from build123d import *

# Parameters (mm, degrees)
SKETCH1_W               = 74.5
SKETCH1_H               = 30
BOSS_EXTRUDE1_DEPTH     = 2
SKETCH4_W               = 2
SKETCH4_H               = 30
BOSS_EXTRUDE2_DEPTH     = 5
CUT_EXTRUDE1_DEPTH      = 41.268629229
CUT_EXTRUDE1_DEPTH_BACK = 41.268629229
SKETCH5_W               = 2
SKETCH5_H               = 15
CUT_EXTRUDE2_DEPTH      = 41.268629229
CUT_EXTRUDE2_DEPTH_BACK = 41.268629229
SKETCH6_R               = 7.5
FILLET1_R               = 1


with BuildPart() as part:
    # Sketch1 → Boss-Extrude1 (new body)
    with BuildSketch(Plane(origin=(0, 0, 0), x_dir=(1, 0, 0), z_dir=(0, 1, 0))):
        Rectangle(SKETCH1_W, SKETCH1_H)
    extrude(amount=BOSS_EXTRUDE1_DEPTH)

    # Sketch4 → Boss-Extrude2 (add)
    with BuildSketch(Plane(origin=(0, 0, 0), x_dir=(1, 0, 0), z_dir=(0, 1, 0))):
        with Locations((36.25, 0)):
            Rectangle(SKETCH4_W, SKETCH4_H)
        with Locations((-36.25, 0)):
            Rectangle(SKETCH4_W, SKETCH4_H)
    extrude(amount=BOSS_EXTRUDE2_DEPTH)

    # Sketch5 → Cut-Extrude1 (cut, two sides: drawn at the far end of the back side and taken through both)
    with BuildSketch(Plane(origin=(0, 2, 0), x_dir=(1, 0, 0), z_dir=(0, 1, 0)).offset(-CUT_EXTRUDE1_DEPTH_BACK)):
        with Locations((0, -7.5)):
            Rectangle(SKETCH5_W, SKETCH5_H)
    extrude(amount=CUT_EXTRUDE1_DEPTH + CUT_EXTRUDE1_DEPTH_BACK, mode=Mode.SUBTRACT)

    # Sketch6 → Cut-Extrude2 (cut, two sides: drawn at the far end of the back side and taken through both)
    with BuildSketch(Plane(origin=(0, 2, 0), x_dir=(1, 0, 0), z_dir=(0, 1, 0)).offset(-CUT_EXTRUDE2_DEPTH_BACK)):
        with Locations((0, 20)):
            Circle(SKETCH6_R)
    extrude(amount=CUT_EXTRUDE2_DEPTH + CUT_EXTRUDE2_DEPTH_BACK, mode=Mode.SUBTRACT)

    # Fillet1
    fillet1_edges = [part.edges().sort_by_distance(p)[0] for p in [
        (1, 1, 15),
        (-1, 1, 15),
        (-1, 1, 0),
        (1, 1, 0),
        (-35.25, 2, 0),
        (35.25, 2, 0),
    ]]
    fillet(fillet1_edges, radius=FILLET1_R - 0.0001)  # a hair under: the kernel refuses the full size


solid = part.part
Geometry: final body of the model. Coordinates: model frame, mm. A direction names the side the tool comes from. Give positions to 0.01 mm unless a question says otherwise; leave off trailing zeros. Write each loop counter-clockwise with the first axis right and the second up, starting at its lowest first coordinate (ties: lowest second). Pieces come first, ordered by that corner, then holes.
(1) Cut plane B-B, the plane y = 4.2. Return loops of the section in (x, z), then the cut area to 3 significant figures.
(2) Cut plane A-A, the plane z = 8. Return loops of the section in (x, y), then the cut area to 3 significant figures.
(3) Access query for faces 1 (the flat face through (1, 1, 8)), 2 (the flat face through (35.25, 4, 0)), 3 (the flat face through (36, 5, 0)). Directions: +Z, -Z, +X, -X, +Y, -Y. A direction counts if a zero-diameter tool reaches every point of the face in a straight line with its end or side. Return the directions, or none.
(4) Ray query, line 1 (Y direction, x = -16, z = -5); line 2 (X direction, y = 2.85, z = -13.5); line 3 (X direction, y = 2.45, z = 6). Return the intervals inside material, ascending.
(5) Mould query, pull axis X, two halves, no side actions, for faces 4 (the cylindrical face through (-0.1, 1, -12.5)), 5 (the flat face through (-1, 0, 0)), 6 (the flat face through (-37.25, 2, 0)). Classes: released by +X, released by -X, zero draft, split by the parting line, or undercut.
(6) First-contact query: P1, Ø12, axis at x = -1, z = 4, coming from the -Y side; P2, Ø5, axis at x = -18.5, z = 7, coming from the +Y side. Flat tips, straight axial feed; report the tip coordinate or a pass-through.
(7) Cut plane D-D, the plane x = -27.5. Return loops of the section in (y, z).
Values follow:
1. outline: (-37.25, -15) - (-35.25, -15) - (-35.25, 15) - (-37.25, 15) - close; (35.25, -15) - (37.25, -15) - (37.25, 15) - (35.25, 15) - close
1. area: 120 mm2
2. outline: (-37.25, 0) - (-1, 0) - (-1, 2) - (-34.25, 2) arc R1 cw to (-35.25, 3) - (-35.25, 5) - (-37.25, 5) - close; (1, 0) - (37.25, 0) - (37.25, 5) - (35.25, 5) - (35.25, 3) arc R1 cw to (34.25, 2) - (1, 2) - close
2. area: 157 mm2
3. face 1: +Z, +Y, -Y
3. face 2: +Z, -Z, +Y
3. face 3: +Z, -Z, +X, -X, +Y
4. line 1: y = 0 to 2
4. line 2: x = -37.25 to -35.24, 35.24 to 37.25
4. line 3: x = -37.25 to -35.09, 35.09 to 37.25
5. face 4: undercut
5. face 5: zero draft
5. face 6: released by -X
6. P1: stops at y = 0
6. P2: stops at y = 2
7. outline: (0, -15) - (2, -15) - (2, 15) - (0, 15) - close
